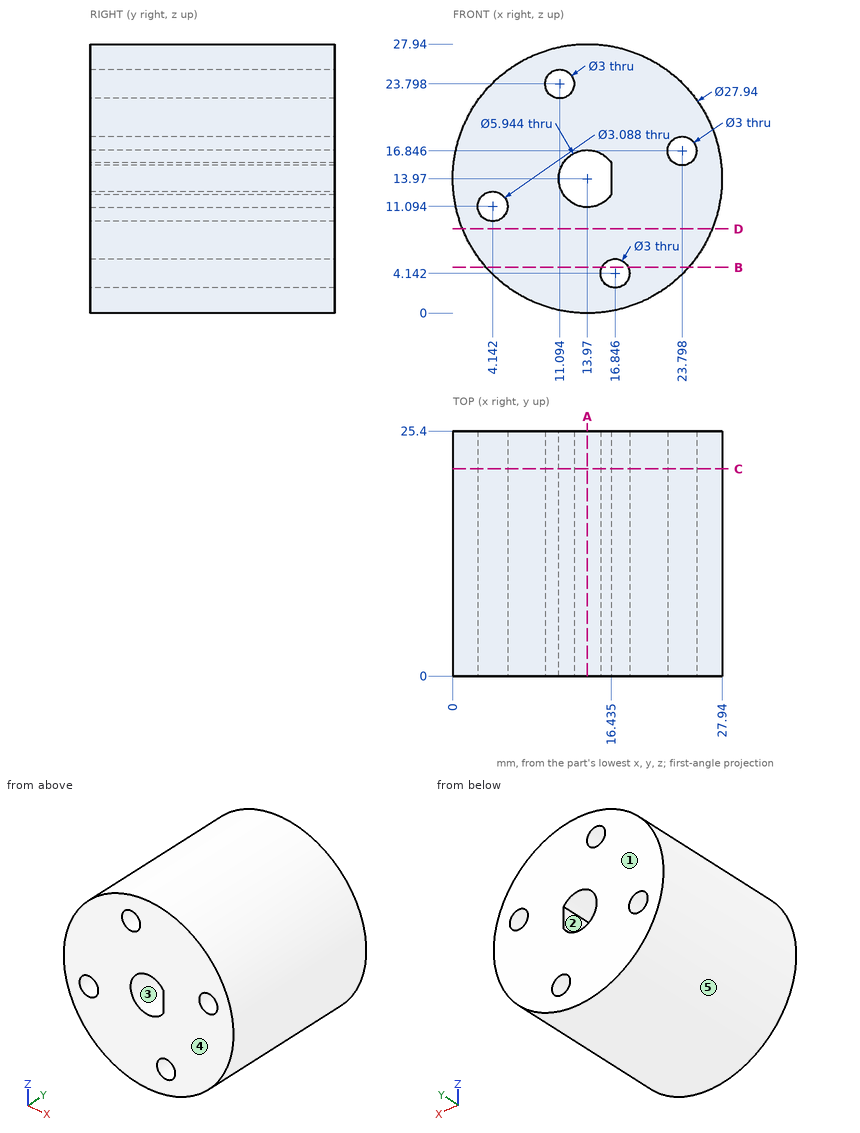
Verification items for this drawing (mm, ordinates from the low corner). A direction names the side the tool comes from. Coordinates: 2 decimals unless noted, no trailing zeros. Write each loop counter-clockwise with the first axis right and the second up, starting at its lowest first coordinate (ties: lowest second). Pieces come first, ordered by that corner, then holes. Notation, with made-up numbers: M 18.25,35.25 L 26.25,35.25 A19 cw 26.25,59.25 Z; hole C 6.5,59.25 d6. An arc over 180 degrees is marked long. Use one line per item in the form item = value. Start each with the question number.
1) Set-up check for the marked faces 1 and 2: record each of +Z, -Z, +X, -X, +Y, -Y from which the full face is reachable in a straight line by a thin tool's end or side.
2) Section check A-A on x = 13.97. Enter the section's corners in (y, z).
3) Thickness scan on probe 1 along X at (y, z) = (4.25, 17.5); probe 2 along Z at (x, y) = (24.5, 11.25); probe 3 along Z at (x, y) = (24, 4.5) (1 decimal). Record the ranges inside material, lowest first. Write a range as from..to.
4) Go/stop test with flat-tipped pins: pin 1 Ø1 at (y, z) = (18.5, 21) entering from +X; pin 2 Ø8 at (y, z) = (7.5, 4) entering from -X; pin 3 Ø3 at (y, z) = (19.5, 20) entering from +X (1 decimal); pin 4 Ø2.5 at (x, z) = (11.09, 23.8) entering from -Y. Record where each tip stops, or that it passes through.
5) Section check B-B on z = 4.75. Enter the section's corners in (x, y) (1 decimal).
6) Section check C-C on y = 21.5. Enter the section's corners in (x, z) (1 decimal).
7) Release check for a two-part mould opening along X. For the marked faces 3, 4 and 5 record: pulls with the +X half, pulls with the -X half, needs draft (parallel to the pull), parting line crosses it, or undercut.
8) Section check D-D on z = 8.75. Enter the section's corners in (x, y), and give its area (3 significant figures).
Responses:
q1.face_1 = +Z, -Z, +X, -X, +Y
q1.face_2 = +Y, -Y
q2.outline = M 0,0 L 25.4,0 L 25.4,11 L 0,11 Z; M 0,16.94 L 25.4,16.94 L 25.4,27.94 L 0,27.94 Z
q3.probe_1 = 0.45..22.45, 25.15..27.49
q3.probe_2 = 4.79..15.52, 18.17..23.15
q3.probe_3 = 4.2..15.4, 18.3..23.7
q4.pin_1 = 26.32
q4.pin_2 = 1.34
q4.pin_3 = 27.2
q4.pin_4 = through
q5.outline = M 3.5,0 L 15.5,0 L 15.5,25.4 L 3.5,25.4 Z; M 18.2,0 L 24.5,0 L 24.5,25.4 L 18.2,25.4 Z
q6.outline = C 14,14 d27.9; hole C 4.1,11.1 d3.1; hole C 11.1,23.8 d3; hole C 16.8,4.1 d3; hole M 16.4,12.3 L 16.4,15.6 A3 ccw long Z; hole C 23.8,16.8 d3
q7.face_3 = undercut
q7.face_4 = needs draft
q7.face_5 = parting line crosses it
q8.outline = M 1.01,0 L 26.93,0 L 26.93,25.4 L 1.01,25.4 Z
q8.area = 658 mm2
